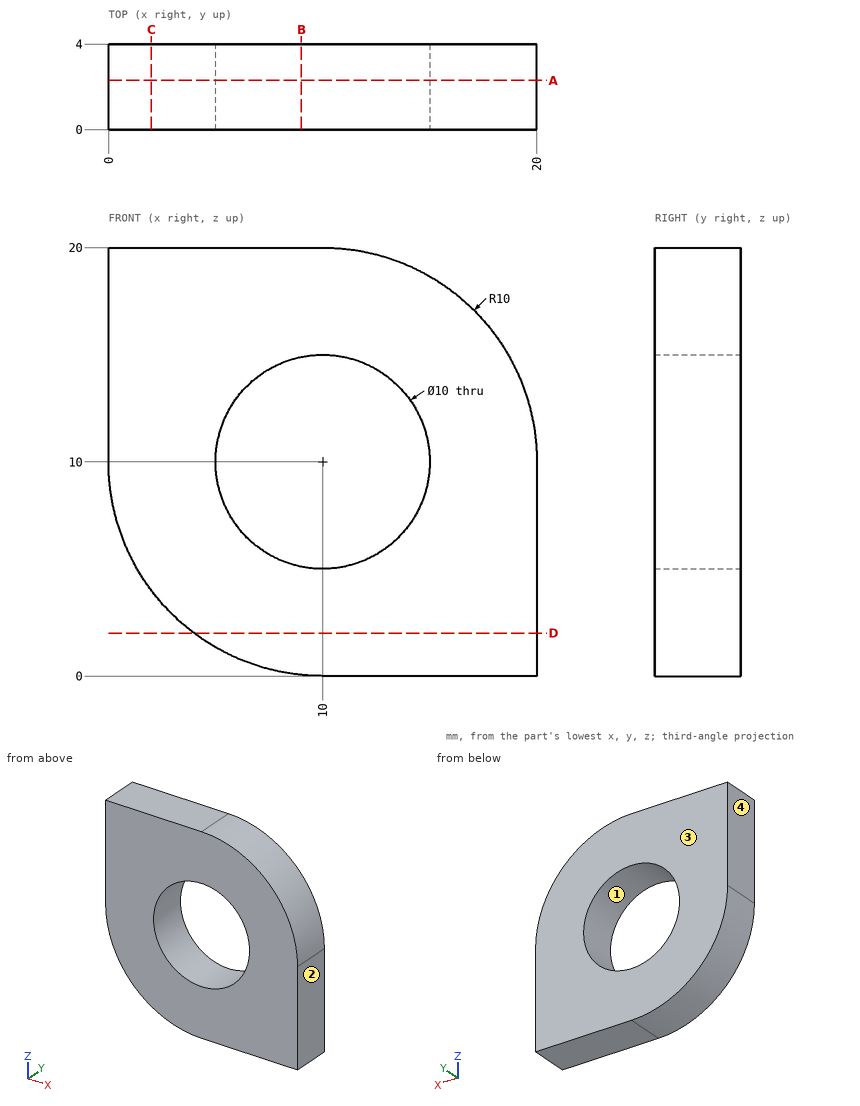
Geometry: see drawing. Coordinates: mm, zero at the bounding-box minimum. Round coordinates to 2 decimals unless told otherwise and drop trailing zeros. Loops run counter-clockwise (first coordinate to the right, second up) from the corner with the lowest first, then second, coordinate; pieces in that order, holes last. Notation, with made-up numbers: M 5,17 L 14,17 A24 ccw 14,55 Z; hole C 80.5,34 d1. An arc over 180 degrees is marked long. Use a Markdown table: item, result. Add a question column.
1. Section query A-A on y = 2.3. Return the cut outline in (x, z), then the cut area to 3 significant figures.
2. Section query B-B on x = 9. Return the cut outline in (y, z).
3. Line query: line 1 (Z direction, x = 10, y = 2.05); line 2 (X direction, y = 0.7, z = 8). Output: solid intervals per line, ascending.
4. Mould query, pull axis X, two halves, no side actions, for the marked faces 1, 2, 3 and 4. Classes: pulls with the +X half, pulls with the -X half, needs draft (parallel to the pull), parting line crosses it, or undercut.
5. Section query D-D on z = 2. Return the cut outline in (x, y), then the cut area to 3 significant figures.
6. Section query C-C on x = 2. Return the cut outline in (y, z), then the cut area to 3 significant figures.
Reported:
| question | item | result |
|---|---|---|
| 1 | outline | M 0,10 A10 ccw 10,0 L 20,0 L 20,10 A10 ccw 10,20 L 0,20 Z; hole C 10,10 d10 |
| 1 | area | 279 mm² |
| 2 | outline | M 0,0.05 L 4,0.05 L 4,5.1 L 0,5.1 Z; M 0,14.9 L 4,14.9 L 4,20 L 0,20 Z |
| 3 | line 1 | z = 0 to 5, 15 to 20 |
| 3 | line 2 | x = 0.2 to 5.42, 14.58 to 20 |
| 4 | face 1 | undercut |
| 4 | face 2 | pulls with the +X half |
| 4 | face 3 | needs draft |
| 4 | face 4 | pulls with the -X half |
| 5 | outline | M 4,0 L 20,0 L 20,4 L 4,4 Z |
| 5 | area | 64.0 mm² |
| 6 | outline | M 0,4 L 4,4 L 4,20 L 0,20 Z |
| 6 | area | 64.0 mm² |
